Design review of the part built by this model. Coordinates are the model's own, in mm. Face numbers are marked on the shaded views. A direction names the side the tool comes from. Coordinates: 2 decimals unless noted, no trailing zeros. Loops run counter-clockwise (first coordinate to the right, second up) from the corner with the lowest first, then second, coordinate; pieces in that order, holes last.
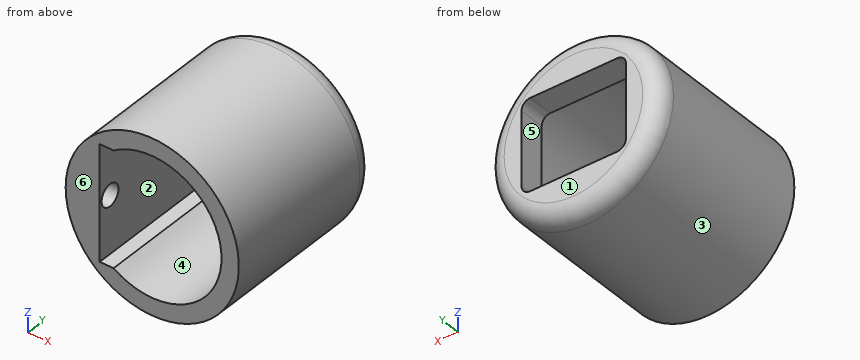
Autodesk Inventor part; units mm, degrees
ref_plane "YZ Plane" through (0, 0, 0) normal (1, 0, 0) x (0, 1, 0)
ref_plane "XZ Plane" through (0, 0, 0) normal (0, 1, 0) x (-1, 0, 0)
ref_plane "XY Plane" through (0, 0, 0) normal (0, 0, 1) x (1, 0, 0)
sketch "Sketch1" plane through (0, 0, 0) normal (0, 1, 0) x (-1, 0, 0)
  circle A0 centre (0, 0) radius 15.875
  dimension "d0" = 31.75
extrude "Extrusion1" add sketch "Sketch1" along normal blind 31.75
fillet "Fillet1" radius 3.175 1 edges at (15.875, 31.75, 0)
sketch "Sketch2" plane through (0, 31.75, 0) normal (0, 1, 0) x (1, 0, 0)
  point P0 (0, 0)
sketch "Sketch3" plane through (0, 0, 0) normal (0, -1, 0) x (1, 0, 0)
  circle A0 centre (0, 0) radius 12.7
  line L0 (-7.091, -10.536) -> (-9.6294, -10.536)
  line L1 (-9.6294, -10.536) -> (-9.6294, 8.2804)
  line L2 (-9.6294, 8.2804) -> (-7.091, 8.2804)
  line L3 (-7.091, 8.2804) -> (-7.091, -10.536)
  line L4 (-7.091, 10.536) -> (-9.6294, 10.536)
  line L5 (-9.6294, 10.536) -> (-9.6294, 8.2804)
  line L6 (-9.6294, 8.2804) -> (-7.091, 8.2804)
  line L7 (-7.091, 8.2804) -> (-7.091, 10.536)
extrude "Extrusion2" cut sketch "Sketch3" against normal blind 26.9875 contours A0 L3 L7 | L7 L2 A0 | A0 L5 L4 | L0 L1 A0 | A0 L1 L2 L3
sketch "Sketch4" plane through (0, 31.75, 0) normal (0, 1, 0) x (1, 0, 0)
  circle A0 centre (0, 0) radius 12.7
  line L0 (-9.6294, 10.536) -> (-9.6294, -10.536)
  line L1 (-9.6294, 8.2804) -> (9.5066, 8.2804)
  line L2 (9.5066, 8.2804) -> (9.5066, -8.4211)
  line L3 (9.5066, -8.4211) -> (-9.6294, -8.4211)
  line L4 (-9.6294, -8.4211) -> (-9.6294, 8.2804)
  point P0 (-9.5066, -8.4211)
  point P1 (-9.6294, -8.2804)
extrude "Extrusion3" cut sketch "Sketch4" against normal blind 4.7625 contours L1 L2 L3 A0 L0
fillet "Fillet2" radius 1.5875 5 edges at (-9.6294, 29.3687, -8.2804) (9.5066, 29.3687, -8.2804) (9.5066, 29.3687, 8.4211) (-9.6294, 29.3687, 8.2804) (-9.5066, 29.3687, 8.4211)
sketch "Sketch5" plane through (-9.6294, 0, 10.536) normal (1, 0, 0) x (0, 0, -1)
  circle A0 centre (10.536, 2.4407) radius 2
  point P0 (10.536, 0)
  dimension "d9" = 4
extrude "Extrusion4" cut sketch "Sketch5" against normal blind 5
properties part number "module"
Q1. For line 1 (Z direction, x = 0, y = 19) (3 decimals); line 2 (Y direction, x = -7, z = 10); line 3 (X direction, y = 6.5, z = 2), list the stretches that pass through material, from the lowest coordinate up.
Q2. The part is to be moulded in two halves that separate along X. For the marked faces 1, 2 and 3, say which applies: pulls with the +X half, pulls with the -X half, needs draft (parallel to the pull), parting line crosses it, or undercut.
Q3. Take a section at D-D, the plane y = 8. Write out the cut boundary in (x, z) (3 decimals), then the cut area to 3 significant figures.
Q4. Machinability: for the marked faces 4, 5 and 6, which of the approach directions +Z, -Z, +X, -X, +Y, -Y give a long, thin tool a straight path to every point of the face, cutting with its end or side? Answer none if there is none.
Q5. Clearance check with flat-ended pins moving along their axes: pin 1 Ø2 at (x, y) = (3, 16) entering from +Z; pin 2 Ø1.4 at (x, y) = (-2.5, 30) entering from -Z; pin 3 Ø2 at (x, y) = (-8, 15.5) entering from -Z. State where each tip first meets the part, or that it passes through.
Q6. Take a section at C-C, the plane y = 3.5. Write out the cut boundary in (x, z) (3 decimals).
Entries:
1. line 1: z = -15.875 to -12.7, 12.7 to 15.875
1. line 2: y = 26.99 to 31.75
1. line 3: x = -15.75 to -9.63, 12.54 to 15.75
2. face 1: needs draft
2. face 2: undercut
2. face 3: parting line crosses it
3. outline: circle Ø31.75 at (0, 0); hole (-9.629, -10.536) - (-7.091, -10.536) arc R12.7 ccw (long way) to (-7.091, 10.536) - (-9.629, 10.536) - close
3. area: 315 mm2
4. face 4: -Y
4. face 5: +Y, -Y
4. face 6: +Z, -Z, +X, -X, -Y
5. pin 1: stops at z = 15.75
5. pin 2: stops at z = -15.62
5. pin 3: stops at z = -14.25
6. outline: circle Ø31.75 at (0, 0); hole (-14.629, -1.696) - (-9.629, -1.696) - (-9.629, -10.536) - (-7.091, -10.536) arc R12.7 ccw (long way) to (-7.091, 10.536) - (-9.629, 10.536) - (-9.629, 1.696) - (-14.629, 1.696) - close
